Autodesk Inventor part; units mm, degrees
ref_plane "YZ Plane" through (0, 0, 0) normal (1, 0, 0) x (0, 1, 0)
ref_plane "XZ Plane" through (0, 0, 0) normal (0, 1, 0) x (-1, 0, 0)
ref_plane "XY Plane" through (0, 0, 0) normal (0, 0, 1) x (1, 0, 0)
sketch "Sketch1" plane through (0, 0, 0) normal (0, 0, 1) x (1, 0, 0)
  line L0 (-10, 56.825) -> (10, 56.825)
  line L1 (10, 56.825) -> (10, -56.825)
  line L2 (10, -56.825) -> (-10, -56.825)
  line L3 (-10, -56.825) -> (-10, 56.825)
  point P0 (0, 0)
  dimension "d0" = 113.65
  dimension "d1" = 56.825
  dimension "d2" = 20
  dimension "d3" = 10
extrude "Extrusion1" add sketch "Sketch1" along normal blind 15
sketch "Sketch2" plane through (0, 0, 15) normal (0, 0, 1) x (1, 0, 0)
  line L0 (-10, -56.825) -> (10, -56.825)
  line L1 (-3.25, 56.825) -> (3.25, 56.825)
  line L2 (3.25, 56.825) -> (3.25, -56.825)
  line L3 (3.25, -56.825) -> (-3.25, -56.825)
  line L4 (-3.25, -56.825) -> (-3.25, 56.825)
  line L5 (-10, 56.825) -> (-10, -56.825)
  line L6 (10, -56.825) -> (10, 56.825)
  point P0 (0, 0)
  dimension "d6" = 6.75
  dimension "d7" = 6.5
  dimension "d8" = 20
extrude "Extrusion2" cut sketch "Sketch2" against normal blind 7.5
equation "\"d6\" = -0.5 * d7 + 0.5 * d8"
properties part number "2208_Back Plate Groove_V1"
The listing builds one solid part. Answer for the finished solid, in the listing's coordinates (mm). A direction names the side the tool comes from. Round coordinates to 2 decimals unless told otherwise and drop trailing zeros. Write each loop counter-clockwise with the first axis right and the second up, starting at its lowest first coordinate (ties: lowest second). Pieces come first, ordered by that corner, then holes. Notation, with made-up numbers: (2, -5.75) - (8, -5.75) arc R14 cw to (8, 12.25) - close; hole circle Ø2 at (-33.75, -32). An arc over 180 degrees is marked (long way). Use a Markdown table: item, result. Add a question column.
1. Flat-ended cylindrical pins translate along their axes: P1, Ø10, axis at x = 4, y = 30, coming from the -Z side; P2, Ø5, axis at x = 0.5, y = 23, coming from the +Z side. Find the tip coordinate at first contact, or state that the pin passes through.
2. The part is cut by section A-A (z = 8.5). Write down the section's boundary in (x, y) (3 decimals).
3. The part is cut by section B-B (y = -38.5). Write down the section's boundary in (x, z), and give its area (3 significant figures).
4. The part is cut by section C-C (x = -0.5). Write down the section's boundary in (y, z) (3 decimals).
5. A tool of negligible diameter and unlimited length cuts with its end or side. For faces 1 (the face through (3.25, 1, 11)), 2 (the face through (0, -56.825, 7)), from which of +Z, -Z, +X, -X, +Y, -Y can it reach the whole face along a straight path? Write none if from no direction.
6. For a pull along X with two mould halves and no side action, classify faces 3 (the face through (-10, -1, 7)), 4 (the face through (7, 1, 15)), 5 (the face through (0, 1, 7.5)) as +X half, -X half, draft (parallel to the pull), parting line (faces both ways), or undercut.
7. Consider line 1 (X direction, y = 35, z = 12.75); line 2 (Z direction, x = -1.75, y = 22.5). Determine where each line is inside the solid, lowest interval first.
Reported:
| question | item | result |
|---|---|---|
| 1 | P1 | z = 0 |
| 1 | P2 | z = 7.5 |
| 2 | outline | (-10, -56.825) - (-3.25, -56.825) - (-3.25, 56.825) - (-10, 56.825) - close; (3.25, -56.825) - (10, -56.825) - (10, 56.825) - (3.25, 56.825) - close |
| 3 | outline | (-10, 0) - (10, 0) - (10, 15) - (3.25, 15) - (3.25, 7.5) - (-3.25, 7.5) - (-3.25, 15) - (-10, 15) - close |
| 3 | area | 251 mm^2 |
| 4 | outline | (-56.825, 0) - (56.825, 0) - (56.825, 7.5) - (-56.825, 7.5) - close |
| 5 | face 1 | +Z, +Y, -Y |
| 5 | face 2 | +Z, -Z, +X, -X, -Y |
| 6 | face 3 | -X half |
| 6 | face 4 | draft |
| 6 | face 5 | undercut |
| 7 | line 1 | -10 to -3.25, 3.25 to 10 |
| 7 | line 2 | 0 to 7.5 |
